The model under review builds one solid part; all positions refer to its coordinate system, in mm. Coordinates: 2 decimals unless noted, no trailing zeros. Loops run counter-clockwise (first coordinate to the right, second up) from the corner with the lowest first, then second, coordinate; pieces in that order, holes last. Notation, with made-up numbers: M 71,49.25 L 91,49.25 A17 ccw 91,79.25 Z; hole C 17,-8 d10. An arc over 180 degrees is marked long. Use CSV: the item, a comma, the result in double quotes. Start each with the question number.
1. For L1, parallel to Y at x = 0.8, z = 37; L2, parallel to Z at x = -1.15, y = -2; L3, parallel to Y at x = -1.9, z = 31, list the stretches that pass through material, from the lowest coordinate up.
2. Add section D-D, the plane z = 33.5. Write out the cut boundary in (x, y), then the cut area to 3 significant figures.
3. Add section C-C, the plane x = 0.9. Write out the cut boundary in (y, z) (3 decimals).
4. Add section B-B, the plane z = 38. Write out the cut boundary in (x, y), then the cut area to 3 significant figures.
5. Clearance check with flat-ended pins moving along their axes: P1, Ø2, axis at x = 0, z = 32.5, coming from the -Y side; P2, Ø5.5, axis at y = 0, z = 37, coming from the +X side; P3, Ø1, axis at x = 0, z = 14.5, coming from the -Y side. State where each tip first meets the part, or that it passes through.
6. Add section A-A, the plane y = 0. Write out the cut boundary in (x, z) (3 decimals), then the cut area to 3 significant figures.
7. Draft analysis for pull direction Y (two halves, no side actions). For faces 1 (the flat face through (0.035, 11.843, 22.256)), 2 (the flat face through (0.04, -11.93, 21.79)), 3 (the cylindrical face through (0, 0, 40)), 4 (the cylindrical face through (0.035, 0.272, 15.873)), state which applies: +Y half, -Y half, draft (parallel to the pull), parting line (faces both ways), or undercut.
from build123d import *

# Parameters (mm, degrees)
SKETCH1_R           = 3
BOSS_EXTRUDE1_DEPTH = 2.5


with BuildPart() as part:
    # Sketch1 → Boss-Extrude1 (new, symmetric)
    with BuildSketch(Plane.YZ):
        with BuildLine():
            Line((-14.917620355, 5.429569775), (-8.85341753, 38.617713829))
            ThreePointArc((-8.85341753, 38.617713829), (0, 46), (8.85341753, 38.617713829))
            Line((8.85341753, 38.617713829), (14.917620355, 5.429569775))
            ThreePointArc((14.917620355, 5.429569775), (0, 15.875), (-14.917620355, 5.429569775))
        make_face()
        with Locations(Location((0, 37, 0), (0, 0, 270))):
            Circle(SKETCH1_R, mode=Mode.SUBTRACT)
    extrude(amount=BOSS_EXTRUDE1_DEPTH, both=True)


solid = part.part
Computed:
1,L1,"y = -9.15 to -3, 3 to 9.15"
1,L2,"z = 15.75 to 34.76, 39.24 to 45.77"
1,L3,"y = -10.25 to 10.25"
2,outline,"M -2.5,-9.79 L 2.5,-9.79 L 2.5,9.79 L -2.5,9.79 Z"
2,area,"97.9 mm^2"
3,outline,"M -14.918,5.43 A15.875 cw 14.918,5.43 L 8.853,38.618 A9 ccw -8.853,38.618 Z; hole C 0,37 d6"
4,outline,"M -2.5,-8.97 L 2.5,-8.97 L 2.5,-2.83 L -2.5,-2.83 Z; M -2.5,2.83 L 2.5,2.83 L 2.5,8.97 L -2.5,8.97 Z"
4,area,"61.4 mm^2"
5,P1,"stops at y = -10.15"
5,P2,"passes through"
5,P3,"stops at y = -13.35"
6,outline,"M -2.5,15.875 L 2.5,15.875 L 2.5,34 L -2.5,34 Z; M -2.5,40 L 2.5,40 L 2.5,46 L -2.5,46 Z"
6,area,"121 mm^2"
7,face 1,"+Y half"
7,face 2,"-Y half"
7,face 3,"undercut"
7,face 4,"undercut"
